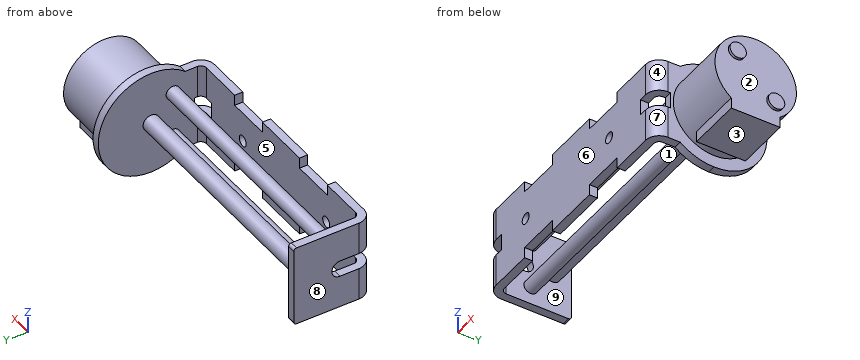
from build123d import *

# Parameters (mm, degrees)
BOSS_EXTRUDE1_DEPTH = 7.5
BOSS_EXTRUDE2_DEPTH = 1.5
SKETCH4_R           = 7.5
BOSS_EXTRUDE3_DEPTH = 12
SKETCH5_R           = 1.5
SKETCH5_R_2         = 1.25
BOSS_EXTRUDE4_DEPTH = 46.5
SKETCH6_R           = 1
CUT_EXTRUDE1_DEPTH  = 1.5
SKETCH7_R           = 1.5
BOSS_EXTRUDE5_DEPTH = 0.5
SKETCH8_W           = 8
SKETCH8_H           = 2
CUT_EXTRUDE2_DEPTH  = 53.627226794
FILLET1_R           = 0.5
SKETCH9_W           = 3
SKETCH9_H           = 3.5
SKETCH9_H_2         = 8.5
CUT_EXTRUDE3_DEPTH  = 4
SKETCH10_W          = 3
SKETCH10_H          = 6
CUT_EXTRUDE4_DEPTH  = 4
SKETCH12_W          = 10
SKETCH12_H          = 9
BOSS_EXTRUDE6_DEPTH = 8


with BuildPart() as part:
    # Sketch1 → Boss-Extrude1 (new, symmetric)
    with BuildSketch(Plane.XY):
        with BuildLine():
            Line((-46.5, 14.5), (-48, 14.5))
            Line((-48, 14.5), (-48, 2.5))
            ThreePointArc((-48, 2.5), (-47.267766953, 0.732233047), (-45.5, 0))
            Line((-45.5, 0), (-2.5, 0))
            ThreePointArc((-2.5, 0), (-0.732233047, 0.732233047), (0, 2.5))
            Line((0, 2.5), (0, 14.5))
            Line((0, 14.5), (-1.5, 14.5))
            Line((-1.5, 14.5), (-1.5, 2.5))
            ThreePointArc((-1.5, 2.5), (-1.792893219, 1.792893219), (-2.5, 1.5))
            Line((-2.5, 1.5), (-45.5, 1.5))
            ThreePointArc((-45.5, 1.5), (-46.207106781, 1.792893219), (-46.5, 2.5))
            Line((-46.5, 2.5), (-46.5, 14.5))
        make_face()
    extrude(amount=BOSS_EXTRUDE1_DEPTH, both=True)

    # Sketch3 → Boss-Extrude2 (add)
    with BuildSketch(Plane(origin=(0, 0, 0), x_dir=(0, 0, -1), z_dir=(1, 0, 0))):
        with BuildLine():
            ThreePointArc((7.5, 4.770032103), (9.170264445, 7.688089675), (9.75, 11))
            ThreePointArc((9.75, 11), (-3.311910325, 20.170264445), (-7.5, 4.770032103))
            Line((-7.5, 4.770032103), (-7.5, 14.5))
            Line((-7.5, 14.5), (7.5, 14.5))
            Line((7.5, 14.5), (7.5, 4.770032103))
        make_face()
    extrude(amount=-BOSS_EXTRUDE2_DEPTH)

    # Sketch4 → Boss-Extrude3 (add)
    with BuildSketch(Plane(origin=(0, 0, 0), x_dir=(0, 0, -1), z_dir=(1, 0, 0))):
        with Locations((0, 11)):
            Circle(SKETCH4_R)
    extrude(amount=BOSS_EXTRUDE3_DEPTH)

    # Sketch5 → Boss-Extrude4 (add)
    with BuildSketch(Plane.ZY.offset(48)):
        with Locations(Location((0, 11, 0), (0, 0, 90))):
            Circle(SKETCH5_R)
        with Locations(Location((4.25, 7, 0), (0, 0, 90))):
            Circle(SKETCH5_R_2)
        with Locations(Location((-4.25, 7, 0), (0, 0, 90))):
            Circle(SKETCH5_R_2)
    extrude(amount=-BOSS_EXTRUDE4_DEPTH)

    # Sketch6 → Cut-Extrude1 (cut)
    with BuildSketch(Plane.XZ):
        with Locations((-37, 0)):
            Circle(SKETCH6_R)
        with Locations((-13, 0)):
            Circle(SKETCH6_R)
    extrude(amount=-CUT_EXTRUDE1_DEPTH, mode=Mode.SUBTRACT)

    # Sketch7 → Boss-Extrude5 (add)
    with BuildSketch(Plane(origin=(12, 0, 0), x_dir=(0, 0, -1), z_dir=(1, 0, 0))):
        with Locations((3.535533906, 14.535533906)):
            Circle(SKETCH7_R)
        with Locations((-3.535533906, 7.464466094)):
            Circle(SKETCH7_R)
    extrude(amount=BOSS_EXTRUDE5_DEPTH)

    # Sketch8 → Cut-Extrude2 (cut, through all)
    with BuildSketch(Plane(origin=(0, 1.5, 0), x_dir=(1, 0, 0), z_dir=(0, 1, 0))):
        with Locations((-33.333333333, -6.5)):
            Rectangle(SKETCH8_W, SKETCH8_H)
        with Locations((-14.666666667, -6.5)):
            Rectangle(SKETCH8_W, SKETCH8_H)
        with Locations((-14.666666667, 6.5)):
            Rectangle(SKETCH8_W, SKETCH8_H)
        with Locations((-33.333333333, 6.5)):
            Rectangle(SKETCH8_W, SKETCH8_H)
    extrude(amount=-CUT_EXTRUDE2_DEPTH, mode=Mode.SUBTRACT)

    # Fillet1
    fillet1_edges = [part.edges().sort_by_distance(p)[0] for p in [
        (-47.25, 14.5, -7.5),
        (-47.25, 14.5, 7.5),
    ]]
    fillet(fillet1_edges, radius=FILLET1_R)

    # Sketch9 → Cut-Extrude3 (cut)
    with BuildSketch(Plane.ZY.offset(48)):
        with BuildLine():
            Line((-1.5, 6), (1.5, 6))
            ThreePointArc((1.5, 6), (0, 7.5), (-1.5, 6))
        make_face()
        with Locations((0, 4.25)):
            Rectangle(SKETCH9_W, SKETCH9_H)
        with Locations((0, -1.75)):
            Rectangle(SKETCH9_W, SKETCH9_H_2)
    extrude(amount=-CUT_EXTRUDE3_DEPTH, mode=Mode.SUBTRACT)

    # Sketch10 → Cut-Extrude4 (cut)
    with BuildSketch(Plane(origin=(0, 0, 0), x_dir=(0, 0, -1), z_dir=(1, 0, 0))):
        Rectangle(SKETCH10_W, SKETCH10_H)
    extrude(amount=-CUT_EXTRUDE4_DEPTH, mode=Mode.SUBTRACT)

    # Sketch12 → Boss-Extrude6 (add)
    with BuildSketch(Plane.XY):
        with Locations((7, 11)):
            Rectangle(SKETCH12_W, SKETCH12_H)
    extrude(amount=-BOSS_EXTRUDE6_DEPTH)


solid = part.part
Check sheet for the modelled part. Datum: model origin and axes. Units: mm. Face numbers are marked on the shaded views. A direction names the side the tool comes from. Round coordinates to 2 decimals unless told otherwise and drop trailing zeros. Write each loop counter-clockwise with the first axis right and the second up, starting at its lowest first coordinate (ties: lowest second). Pieces come first, ordered by that corner, then holes. Notation, with made-up numbers: (-19, 42.5) -> (-14, 42.5) arc R28 ccw to (-14, 63.5) -> close; hole circle Ø4 at (75.5, -3.5). An arc over 180 degrees is marked (long way). Answer as CSV lines item,"result". Start each with the question number.
1) Release check for a two-part mould opening along X. For the marked faces 6, 7, 8 and 9 record: pulls with the +X half, pulls with the -X half, needs draft (parallel to the pull), parting line crosses it, or undercut.
2) Section check C-C on x = -26. Enter the section's corners in (y, z), and give its area (3 significant figures).
3) Section check A-A on x = -13. Enter the section's corners in (y, z), and give its area (3 significant figures).
4) Section check B-B on z = 0. Enter the section's corners in (x, y).
5) Section check D-D on y = 19.75. Enter the section's corners in (x, z), and give its area (3 significant figures).
6) Go/stop test with flat-tipped pins: P1, Ø10, axis at x = -13, y = 3, coming from the +Z side; P2, Ø4.5, axis at x = -17.5, z = 1.5, coming from the +Y side; P3, Ø1.2, axis at y = 1, z = 7, coming from the +X side. Record where each tip stops, or that it passes through.
7) Tool access check on the marked faces 1, 2, 3, 4 and 5. Record the directions out of +Z, -Z, +X, -X, +Y, -Y that give a thin tool (end or side, any length) a straight path to the whole face; none if there is none.
8) Material ranges on line 1 (X direction, y = 3.75, z = -5.75); line 2 (Z direction, x = -13, y = 0.65); line 3 (X direction, y = 12, z = -7.25), recorded low to high. Write a range as from..to.
Found:
1,face 6,"needs draft"
1,face 7,"pulls with the +X half"
1,face 8,"pulls with the -X half"
1,face 9,"undercut"
2,outline,"(0, -7.5) -> (1.5, -7.5) -> (1.5, 7.5) -> (0, 7.5) -> close; circle Ø2.5 at (7, -4.25); circle Ø2.5 at (7, 4.25); circle Ø3 at (11, 0)"
2,area,"39.4 mm^2"
3,outline,"(0, -5.5) -> (1.5, -5.5) -> (1.5, -1) -> (0, -1) -> close; (0, 1) -> (1.5, 1) -> (1.5, 5.5) -> (0, 5.5) -> close; circle Ø2.5 at (7, -4.25); circle Ø2.5 at (7, 4.25); circle Ø3 at (11, 0)"
3,area,"30.4 mm^2"
4,outline,"(-48, 7.5) -> (-46.5, 7.5) -> (-46.5, 9.5) -> (-1.5, 9.5) -> (-1.5, 3) -> (0, 3) -> (0, 3.5) -> (12, 3.5) -> (12, 18.5) -> (0, 18.5) -> (0, 20.75) -> (-1.5, 20.75) -> (-1.5, 12.5) -> (-46.5, 12.5) -> (-46.5, 14.5) -> (-48, 14.5) -> close; (-44, 0) -> (-38, 0) -> (-38, 1.5) -> (-44, 1.5) -> close; (-36, 0) -> (-14, 0) -> (-14, 1.5) -> (-36, 1.5) -> close; (-12, 0) -> (-4, 0) -> (-4, 1.5) -> (-12, 1.5) -> close"
5,outline,"(-1.5, -4.3) -> (0, -4.3) -> (0, 4.3) -> (-1.5, 4.3) -> close"
5,area,"12.9 mm^2"
6,P1,"stops at z = 7.5"
6,P2,"stops at y = 12.5"
6,P3,"stops at x = -0.17"
7,face 1,"none"
7,face 2,"+X"
7,face 3,"-Z, +X, +Y, -Y"
7,face 4,"+Z, -Z, +X, -Y"
7,face 5,"+Z, -Z"
8,line 1,"x = -48..-46.5, -1.5..0"
8,line 2,"z = -5.5..-1, 1..5.5"
8,line 3,"x = -48..-46.5, -1.5..12"
